Geometry: final body of the model. Coordinates: model frame, mm. A direction names the side the tool comes from. Coordinates: 2 decimals unless noted, no trailing zeros. Loops run counter-clockwise (first coordinate to the right, second up) from the corner with the lowest first, then second, coordinate; pieces in that order, holes last. Notation, with made-up numbers: (-21, 20.5) -> (10, 20.5) arc R21 cw to (10, 44.5) -> close; hole circle Ø7 at (53.25, 51). An arc over 180 degrees is marked (long way). One line per item, written item: value. Start each with the question number.
Item 1: Section query B-B on x = 0. Return loops of the section in (y, z).
Item 2: Contact query for flat-ended pins moving along their axis: pin 1 Ø10 at (x, y) = (28.5, -13) entering from +Z; pin 2 Ø1.8 at (x, y) = (-51, -28.5) entering from +Z; pin 3 Ø3.5 at (x, y) = (56.5, 39) entering from +Z. Output: stop coordinate, or through.
Item 3: Ray query, probe 1 along Y at (x, z) = (-56.5, 36.65); probe 2 along Y at (x, z) = (-21.67, 6); probe 3 along Y at (x, z) = (46, 37.5). Return the intervals inside material, ascending. Write a range as from..to.
Item 4: Mould query, pull axis X, two halves, no side actions, for faces 5 (the cylindrical face through (-60.789, -43.196, 20.28)), 6 (the flat face through (-1, 1, 0)), 7 (the flat face through (1, 41, 22)). Classes: +X half, -X half, draft (parallel to the pull), parting line (faces both ways), or undercut.
Item 5: Section query A-A on y = 0. Return loops of the section in (x, z), then the cut area to 3 significant figures.
Item 6: Section query C-C on y = -19. Return loops of the section in (x, z).
Item 7: Set-up query: faces 1 (the conical face through (55.26, 38.05, 23.37)), 2 (the cylindrical face through (-44.4, 0, 2)), 3 (the cylindrical face through (60.789, 43.196, 20.28)), 4 (the cylindrical face through (-22.86, 28.32, 5.2)). Return all of +Z, -Z, +X, -X, +Y, -Y with unobstructed straight access to the full face (end or side cutting, diameter ignored); none if empty.
Item 8: Section query D-D on x = 40. Return loops of the section in (y, z), then the cut area to 3 significant figures.
from build123d import *

# Parameters (mm, degrees)
SKETCH1_W                               = 125
SKETCH1_H                               = 90
BOSS_EXTRUDE1_DEPTH                     = 40
FILLET1_R                               = 6
CBORE_FOR_M5_HEX_HEAD_BOLT1_D           = 3
CBORE_FOR_M5_HEX_HEAD_BOLT1_DEPTH       = 12
CBORE_FOR_M5_HEX_HEAD_BOLT1_CBORE_D     = 4.2
CBORE_FOR_M5_HEX_HEAD_BOLT1_CBORE_DEPTH = 5
CBORE_FOR_M5_HEX_HEAD_BOLT1_TIP         = 0.901290929
SHELL2_START                            = 4
SHELL2_DEPTH                            = 36
SHELL2_2_DEPTH                          = 21.736908887
SHELL2_START_2                          = 23.633896721
SHELL2_3_DEPTH                          = 7.366103279
SKETCH7_R                               = 3
BOSS_EXTRUDE2_DEPTH                     = 5
M3X0_5_TAPPED_HOLE1_D                   = 2.5
M3X0_5_TAPPED_HOLE1_DEPTH               = 7.5
M3X0_5_TAPPED_HOLE1_TIP                 = 0.751075774
CUT_EXTRUDE1_DEPTH                      = 86.013234264
SKETCH7_5_R                             = 5
CUT_EXTRUDE2_DEPTH                      = 86.013234264
CUT_EXTRUDE3_DEPTH                      = 86.013234264


with BuildPart() as part:
    # Sketch1 → Boss-Extrude1 (new body)
    with BuildSketch(Plane.XY):
        Rectangle(SKETCH1_W, SKETCH1_H)
    extrude(amount=BOSS_EXTRUDE1_DEPTH)

    # Fillet1
    fillet1_edges = [part.edges().sort_by_distance(p)[0] for p in [
        (62.5, -45, 20),
        (-62.5, -45, 20),
        (-62.5, 45, 20),
        (62.5, 45, 20),
    ]]
    fillet(fillet1_edges, radius=FILLET1_R)

    # CBORE for M5 Hex Head Bolt1
    with Locations(Plane.XY.offset(40)):
        with Locations((-56.5, 39), (56.5, 39), (56.5, -39), (-56.5, -39)):
            CounterBoreHole(CBORE_FOR_M5_HEX_HEAD_BOLT1_D / 2, CBORE_FOR_M5_HEX_HEAD_BOLT1_CBORE_D / 2, CBORE_FOR_M5_HEX_HEAD_BOLT1_CBORE_DEPTH, depth=CBORE_FOR_M5_HEX_HEAD_BOLT1_DEPTH)
            with Locations((0, 0, -(CBORE_FOR_M5_HEX_HEAD_BOLT1_DEPTH + CBORE_FOR_M5_HEX_HEAD_BOLT1_TIP / 2))):  # 118° drill point
                Cone(0, CBORE_FOR_M5_HEX_HEAD_BOLT1_D / 2, CBORE_FOR_M5_HEX_HEAD_BOLT1_TIP, mode=Mode.SUBTRACT)

    # Shell2: read off the stored shape, not the designer's step
    # Shell2 outline → Shell2 (cut)
    with BuildSketch(Plane.XY.offset(SHELL2_START)):
        with BuildLine():
            ThreePointArc((58.5, 33.237188186), (52.186648635, 34.686648635), (50.737188186, 41))
            Line((50.737188186, 41), (-50.737188186, 41))
            ThreePointArc((-50.737188186, 41), (-52.186648635, 34.686648635), (-58.5, 33.237188186))
            Line((-58.5, 33.237188186), (-58.5, -33.237188186))
            ThreePointArc((-58.5, -33.237188186), (-52.186648635, -34.686648635), (-50.737188186, -41))
            Line((-50.737188186, -41), (50.737188186, -41))
            ThreePointArc((50.737188186, -41), (52.186648635, -34.686648635), (58.5, -33.237188186))
            Line((58.5, -33.237188186), (58.5, 33.237188186))
        make_face()
    extrude(amount=SHELL2_DEPTH, mode=Mode.SUBTRACT)

    # Shell2 2 outline → Shell2 2 (cut)
    with BuildSketch(Plane.XY.offset(SHELL2_START)):
        with BuildLine():
            Line((56.5, 41), (50.737188186, 41))
            ThreePointArc((50.737188186, 41), (52.186648635, 34.686648635), (58.5, 33.237188186))
            Line((58.5, 33.237188186), (58.5, 39))
            ThreePointArc((58.5, 39), (57.914213562, 40.414213562), (56.5, 41))
        make_face()
        with BuildLine():
            ThreePointArc((-58.5, 33.237188186), (-52.186648635, 34.686648635), (-50.737188186, 41))
            Line((-50.737188186, 41), (-56.5, 41))
            ThreePointArc((-56.5, 41), (-57.914213562, 40.414213562), (-58.5, 39))
            Line((-58.5, 39), (-58.5, 33.237188186))
        make_face()
        with BuildLine():
            ThreePointArc((58.5, -33.237188186), (52.186648635, -34.686648635), (50.737188186, -41))
            Line((50.737188186, -41), (56.5, -41))
            ThreePointArc((56.5, -41), (57.914213562, -40.414213562), (58.5, -39))
            Line((58.5, -39), (58.5, -33.237188186))
        make_face()
        with BuildLine():
            ThreePointArc((-50.737188186, -41), (-52.186648635, -34.686648635), (-58.5, -33.237188186))
            Line((-58.5, -33.237188186), (-58.5, -39))
            ThreePointArc((-58.5, -39), (-57.914213562, -40.414213562), (-56.5, -41))
            Line((-56.5, -41), (-50.737188186, -41))
        make_face()
    extrude(amount=SHELL2_2_DEPTH, mode=Mode.SUBTRACT)

    # Shell2 3 outline → Shell2 3 (cut)
    with BuildSketch(Plane.XY.offset(SHELL2_START_2)):
        with BuildLine():
            ThreePointArc((58.5, 33.876524617), (52.610912703, 35.110912703), (51.376524617, 41))
            Line((51.376524617, 41), (50.737188186, 41))
            ThreePointArc((50.737188186, 41), (52.186648635, 34.686648635), (58.5, 33.237188186))
            Line((58.5, 33.237188186), (58.5, 33.876524617))
        make_face()
        with BuildLine():
            ThreePointArc((-58.5, 33.237188186), (-52.186648635, 34.686648635), (-50.737188186, 41))
            Line((-50.737188186, 41), (-51.376524617, 41))
            ThreePointArc((-51.376524617, 41), (-52.610912703, 35.110912703), (-58.5, 33.876524617))
            Line((-58.5, 33.876524617), (-58.5, 33.237188186))
        make_face()
        with BuildLine():
            Line((58.5, -33.876524617), (58.5, -33.237188186))
            ThreePointArc((58.5, -33.237188186), (52.186648635, -34.686648635), (50.737188186, -41))
            Line((50.737188186, -41), (51.376524617, -41))
            ThreePointArc((51.376524617, -41), (52.610912703, -35.110912703), (58.5, -33.876524617))
        make_face()
        with BuildLine():
            ThreePointArc((-50.737188186, -41), (-52.186648635, -34.686648635), (-58.5, -33.237188186))
            Line((-58.5, -33.237188186), (-58.5, -33.876524617))
            ThreePointArc((-58.5, -33.876524617), (-52.610912703, -35.110912703), (-51.376524617, -41))
            Line((-51.376524617, -41), (-50.737188186, -41))
        make_face()
    extrude(amount=SHELL2_3_DEPTH, mode=Mode.SUBTRACT)

    # Shell2 4 outline → Shell2 4 (revolve)
    with BuildSketch(Plane(origin=(56.5, 39, 0), x_dir=(1, 0, 0), z_dir=(0, -1, 0))):
        Polygon((0, 25.736908889), (0, 22.432175483), (5.500000002, 25.736908889), align=None)
    revolve(axis=Axis((56.5, 39, 0), (0, 0, 1)))

    # Shell2 5 outline → Shell2 5 (revolve)
    with BuildSketch(Plane(origin=(56.5, -39, 0), x_dir=(1, 0, 0), z_dir=(0, -1, 0))):
        Polygon((0, 25.736908889), (0, 22.432175483), (5.500000002, 25.736908889), align=None)
    revolve(axis=Axis((56.5, -39, 0), (0, 0, 1)))

    # Shell2 6 outline → Shell2 6 (revolve)
    with BuildSketch(Plane(origin=(-56.5, 39, 0), x_dir=(1, 0, 0), z_dir=(0, -1, 0))):
        Polygon((0, 25.736908889), (0, 22.432175483), (5.500000002, 25.736908889), align=None)
    revolve(axis=Axis((-56.5, 39, 0), (0, 0, 1)))

    # Shell2 7 outline → Shell2 7 (revolve)
    with BuildSketch(Plane(origin=(-56.5, -39, 0), x_dir=(1, 0, 0), z_dir=(0, -1, 0))):
        Polygon((0, 25.736908887), (0, 22.432175483), (5.5, 25.736908887), align=None)
    revolve(axis=Axis((-56.5, -39, 0), (0, 0, 1)))

    # Sketch7 → Boss-Extrude2 (add)
    with BuildSketch(Plane.XY.offset(4)):
        with Locations((-52.15, 27.94)):
            Circle(SKETCH7_R)
        with Locations((-21.67, 27.94)):
            Circle(SKETCH7_R)
        with Locations((-52.15, -27.94)):
            Circle(SKETCH7_R)
        with Locations((-21.67, -27.94)):
            Circle(SKETCH7_R)
    extrude(amount=BOSS_EXTRUDE2_DEPTH)

    # M3x0.5 Tapped Hole1
    with Locations(Plane.XY.offset(9)):
        with Locations((-52.15, 27.94), (-21.67, 27.94), (-21.67, -27.94), (-52.15, -27.94)):
            Hole(M3X0_5_TAPPED_HOLE1_D / 2, depth=M3X0_5_TAPPED_HOLE1_DEPTH)
            with Locations((0, 0, -(M3X0_5_TAPPED_HOLE1_DEPTH + M3X0_5_TAPPED_HOLE1_TIP / 2))):  # 118° drill point
                Cone(0, M3X0_5_TAPPED_HOLE1_D / 2, M3X0_5_TAPPED_HOLE1_TIP, mode=Mode.SUBTRACT)

    # Sketch7<4> → Cut-Extrude1 (cut, through all)
    with BuildSketch(Plane.XY.offset(4)):
        with BuildLine():
            Line((-52.15, 1.75), (-46.15, 1.75))
            ThreePointArc((-46.15, 1.75), (-44.4, 0), (-46.15, -1.75))
            Line((-46.15, -1.75), (-52.15, -1.75))
            ThreePointArc((-52.15, -1.75), (-53.9, 0), (-52.15, 1.75))
        make_face()
    extrude(amount=-CUT_EXTRUDE1_DEPTH, mode=Mode.SUBTRACT)

    # Sketch7<5> → Cut-Extrude2 (cut, through all)
    with BuildSketch(Plane.XY.offset(4)):
        with Locations((0, -27.94)):
            Circle(SKETCH7_5_R)
    extrude(amount=-CUT_EXTRUDE2_DEPTH, mode=Mode.SUBTRACT)

    # Sketch7<6> → Cut-Extrude3 (cut, through all)
    with BuildSketch(Plane.XY.offset(4)):
        with BuildLine():
            Line((53.9, 3), (53.9, -3))
            ThreePointArc((53.9, -3), (52.15, -4.75), (50.4, -3))
            Line((50.4, -3), (50.4, 3))
            ThreePointArc((50.4, 3), (52.15, 4.75), (53.9, 3))
        make_face()
    extrude(amount=-CUT_EXTRUDE3_DEPTH, mode=Mode.SUBTRACT)


solid = part.part
Reply:
1. outline: (-45, 0) -> (-32.94, 0) -> (-32.94, 4) -> (-41, 4) -> (-41, 40) -> (-45, 40) -> close; (-22.94, 0) -> (45, 0) -> (45, 40) -> (41, 40) -> (41, 4) -> (-22.94, 4) -> close
2. pin 1: stops at z = 4
2. pin 2: stops at z = 9
2. pin 3: stops at z = 35
3. probe 1: y = -45..-41.1, -36.9..-32.9, 32.9..36.9, 41.1..45
3. probe 2: y = -45..-41, -30.94..-29.19, -26.69..-24.94, 24.94..26.69, 29.19..30.94, 41..45
3. probe 3: y = -45..-41, 41..45
4. face 5: -X half
4. face 6: draft
4. face 7: undercut
5. outline: (-62.5, 0) -> (-53.9, 0) -> (-53.9, 4) -> (-58.5, 4) -> (-58.5, 40) -> (-62.5, 40) -> close; (-44.4, 0) -> (50.4, 0) -> (50.4, 4) -> (-44.4, 4) -> close; (53.9, 0) -> (62.5, 0) -> (62.5, 40) -> (58.5, 40) -> (58.5, 4) -> (53.9, 4) -> close
5. area: 736 mm²
6. outline: (-62.5, 0) -> (62.5, 0) -> (62.5, 40) -> (58.5, 40) -> (58.5, 4) -> (-58.5, 4) -> (-58.5, 40) -> (-62.5, 40) -> close
7. face 1: none
7. face 2: +Z, -Z
7. face 3: +Z, -Z, +X, +Y
7. face 4: +Z
8. outline: (-45, 0) -> (45, 0) -> (45, 40) -> (41, 40) -> (41, 4) -> (-41, 4) -> (-41, 40) -> (-45, 40) -> close
8. area: 648 mm²
